Verification items for the finished model (mm, model axes). Coordinates: 2 decimals unless noted, no trailing zeros. Write each loop counter-clockwise with the first axis right and the second up, starting at its lowest first coordinate (ties: lowest second). Pieces come first, ordered by that corner, then holes. Notation, with made-up numbers: M -35.5,41.5 L 11.5,41.5 A29 ccw 11.5,61.5 Z; hole C 78.5,-24.75 d4. An arc over 180 degrees is marked long. Answer in a Markdown table with one row per item.
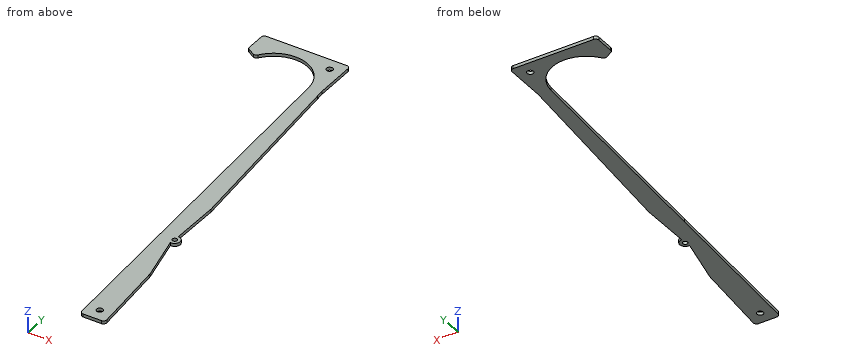
Autodesk Inventor part; units mm, degrees
ref_plane "YZ Plane" through (0, 0, 0) normal (1, 0, 0) x (0, 1, 0)
ref_plane "XZ Plane" through (0, 0, 0) normal (0, 1, 0) x (-1, 0, 0)
ref_plane "XY Plane" through (0, 0, 0) normal (0, 0, 1) x (1, 0, 0)
sketch "Sketch1" plane through (0, 0, 0) normal (0, 0, 1) x (1, 0, 0)
  line L0 (82.55, -393.7) -> (48.2795, -5.3201)
  line L1 (47.853, -228.6) -> (34.8698, 1.9636)
  line L2 (57.15, -393.7) -> (82.55, -393.7)
  circle A0 centre (69.155, -381) radius 3.175
  line L3 (0, 0) -> (-58.2409, 0) construction
  line L4 (-30.2459, 17.4625) -> (-41.2445, 23.8125)
  line L5 (47.5493, 47.625) -> (47.5493, 2.9548)
  arc A1 (34.8698, 1.9636) -> (-30.2459, 17.4625) centre (0, 0) ccw
  line L6 (-41.2445, 47.625) -> (-41.2445, 23.8125)
  line L7 (-41.2445, 47.625) -> (161.9555, 47.625) construction
  line L8 (-41.2445, 47.625) -> (161.9555, 47.625) construction
  line L9 (-41.2445, 47.625) -> (161.9555, 47.625) construction
  line L10 (-41.2445, 47.625) -> (161.9555, 47.625) construction
  line L11 (-41.2445, 47.625) -> (47.5493, 47.625)
  line L12 (47.853, -228.6) -> (57.15, -393.7)
  circle A2 centre (64.77, -255.905) radius 2.3813
  circle A3 centre (34.8493, 34.925) radius 3.175
  circle A4 centre (64.77, -255.905) radius 5.5993
  line L13 (64.7552, -250.3058) -> (65.4147, -199.51)
  line L14 (63.8836, -261.4336) -> (75.2478, -310.9462)
  line L15 (75.2478, -310.9462) -> (65.4147, -199.51)
  line L16 (48.2795, -5.3201) -> (47.5493, 2.9548)
  point P0 (47.5493, 25.2899)
  point P1 (51.4288, -292.1)
  point P2 (66.5391, -212.2523)
  point P3 (73.9365, -296.0849)
  dimension "d0" = 69.85
  dimension "d1" = 30
  dimension "d2" = 57.15
  dimension "d3" = 25.4
  dimension "d4" = 393.7
  dimension "d5" = 6.35
  dimension "d6" = 12.7
  dimension "d7" = 12.7
  dimension "d8" = 4.7625
  dimension "d9" = 7.62
  dimension "d10" = 137.795
  dimension "d11" = 6.35
  dimension "d12" = 12.7
  dimension "d13" = 12.7
  dimension "d23" = 50.8
  dimension "d24" = 50.8
extrude "Extrusion4" add sketch "Sketch1" along normal blind 3.175 contours L2 L12 L1 A1 L4 L6 L11 L5 L16 L0 L13 A4 L14 | A4
fillet "Fillet1" radius 3.175 6 edges at (-30.2459, 17.4625, 1.5875) (47.5493, 47.625, 1.5875) (-41.2445, 47.625, 1.5875) (82.55, -393.7, 1.5875) (57.15, -393.7, 1.5875) (-41.2445, 23.8125, 1.5875)
sketch "Sketch2" plane through (0, 0, 3.175) normal (0, 0, 1) x (1, 0, 0)
  arc A0 (-41.2445, 25.6456) -> (-39.657, 22.896) centre (-38.0695, 25.6456) ccw
  line L0 (-39.657, 22.896) -> (-32.8808, 18.9837)
  arc A1 (-32.8808, 18.9837) -> (-28.6855, 19.9223) centre (-31.2933, 21.7334) ccw
  arc A2 (34.8698, 1.9636) -> (-28.6855, 19.9223) centre (0, 0) ccw
  line L1 (34.8698, 1.9636) -> (56.9813, -390.7035)
  arc A3 (56.9813, -390.7035) -> (60.1512, -393.7) centre (60.1512, -390.525) ccw
  line L2 (60.1512, -393.7) -> (79.0825, -393.7)
  arc A4 (79.0825, -393.7) -> (82.2452, -390.2459) centre (79.0825, -390.525) ccw
  line L3 (82.2452, -390.2459) -> (75.2478, -310.9462)
  line L4 (75.2478, -310.9462) -> (63.8836, -261.4336)
  arc A5 (63.8836, -261.4336) -> (64.7552, -250.3058) centre (64.77, -255.905) ccw
  line L5 (64.7552, -250.3058) -> (65.4147, -199.51)
  line L6 (65.4147, -199.51) -> (47.5493, 2.9548)
  line L7 (47.5493, 2.9548) -> (47.5493, 44.45)
  arc A6 (47.5493, 44.45) -> (44.3743, 47.625) centre (44.3743, 44.45) ccw
  line L8 (44.3743, 47.625) -> (-38.0695, 47.625)
  arc A7 (-38.0695, 47.625) -> (-41.2445, 44.45) centre (-38.0695, 44.45) ccw
  line L9 (-41.2445, 44.45) -> (-41.2445, 25.6456)
  circle A8 centre (69.155, -381) radius 3.175
  circle A9 centre (34.8493, 34.925) radius 3.175
  circle A10 centre (64.77, -255.905) radius 2.3813
  arc A11 (36.6934, -30.4217) -> (-30.6002, 18.635) centre (-17.0402, -33.4475) ccw
  line L10 (38.8613, -68.9195) -> (6.8988, -20.7299)
  dimension "d30" = 30.332
properties part number "PassiveHooks3"
1) Thickness scan on L1, parallel to X at y = -381, z = 0.7; L2, parallel to X at y = -252.5, z = 2.8; L3, parallel to Y at x = 3, z = 2.55 (3 decimals). Record the ranges inside material, lowest first. Write a range as [from, to].
Response values:
| item | result |
|---|---|
| L1 | x = [56.43, 65.98], [72.33, 81.43] |
| L2 | x = [49.2, 69.22] |
| L3 | y = [34.796, 47.625] |
2) Sectioned sample at B-B (x = -24). Record the cut outline in (y, z) (3 decimals).
Response values:
| item | result |
|---|---|
| outline | M 25.372,0 L 47.625,0 L 47.625,3.175 L 25.372,3.175 Z |
3) Depth check by flat-ended pin: pin 1 (1 mm diameter, centred on y = -55.5, z = 2, fed in from +X); pin 2 (1.6 mm diameter, centred on y = 25, z = 2, fed in from +X). Enter the tip coordinate at first touch or a pass-through.
Response values:
| item | result |
|---|---|
| pin 1 | stops at x = 52.75 |
| pin 2 | stops at x = 47.55 |
4) Sectioned sample at C-C (y = -104). Record the cut outline in (x, z) (3 decimals).
Response values:
| item | result |
|---|---|
| outline | M 40.837,0 L 56.987,0 L 56.987,3.175 L 40.837,3.175 Z |
5) Sectioned sample at A-A (z = 2.1). Give the number of separate pieces and of enclosed holes in the cut face, then the cut area to 3 significant figures.
Response values:
| item | result |
|---|---|
| separate pieces | 1 |
| enclosed holes | 3 |
| area | 9,260 mm² |
